Geometry check sheet. Reference: drawing and pictorial views, mm from the part's lowest x, y, z. Give positions to 0.01 mm unless a question says otherwise; leave off trailing zeros. Order: outer loops, then holes, each group sorted by start corner. A loop starts at its lowest first (then second) coordinate and runs counter-clockwise, first axis right, second up. Notation, with made-up numbers: M 68,89.25 L 110,89.25 A12 cw 110,110.25 Z; hole C 2.25,14 d3. An arc over 180 degrees is marked long. Answer as CSV lines item,"result".
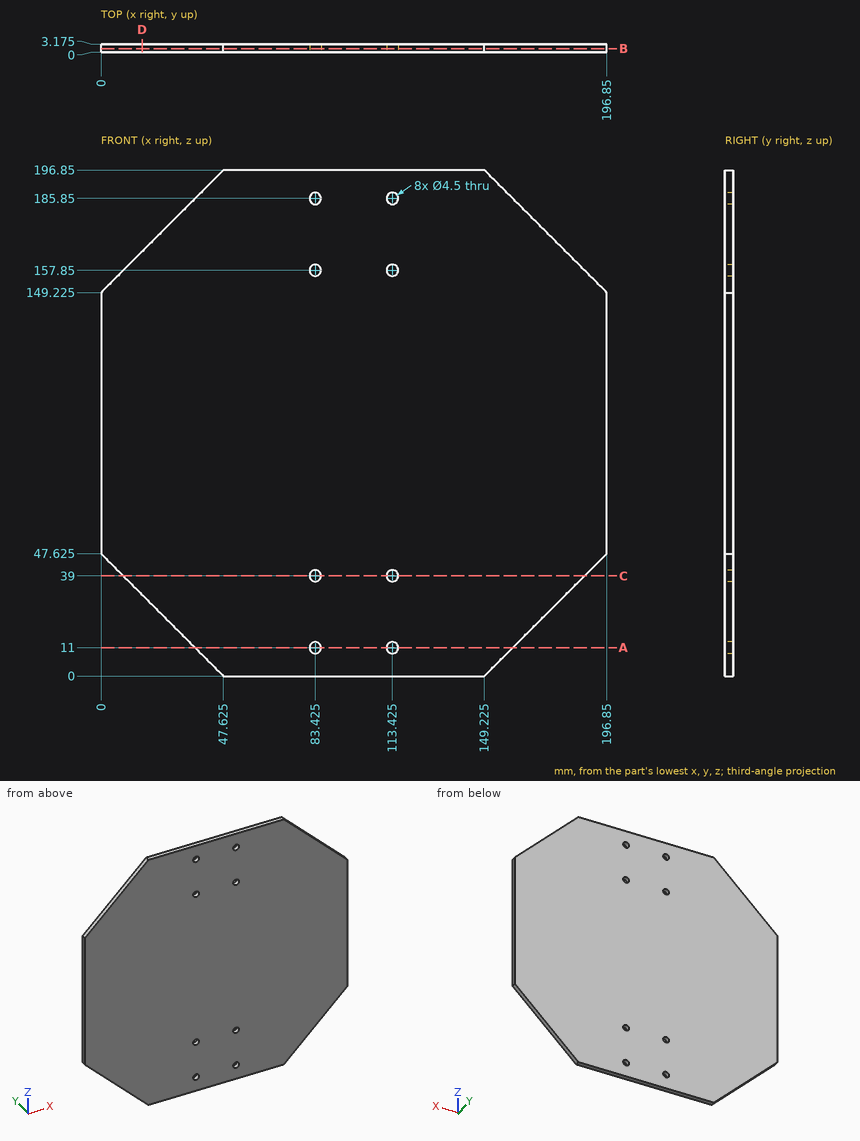
(1) Section check C-C on z = 39. Enter the section's corners in (x, y) (3 decimals).
The answers:
outline,"M 8.625,0 L 81.175,0 L 81.175,3.175 L 8.625,3.175 Z; M 85.675,0 L 111.175,0 L 111.175,3.175 L 85.675,3.175 Z; M 115.675,0 L 188.225,0 L 188.225,3.175 L 115.675,3.175 Z"
(2) Material ranges on line 1 (X direction, y = 1.6, z = 39) (3 decimals); line 2 (Z direction, x = 159, y = 1.9) (3 decimals); line 3 (Z direction, x = 32, y = 0.9) (3 decimals), recorded low to high.
The answers:
line 1,"x = 8.625 to 81.175, 85.675 to 111.175, 115.675 to 188.225"
line 2,"z = 9.775 to 187.075"
line 3,"z = 15.625 to 181.225"
(3) Section check A-A on z = 11. Enter the section's corners in (x, y) (3 decimals), then the cut area to 3 significant figures.
The answers:
outline,"M 36.625,0 L 81.175,0 L 81.175,3.175 L 36.625,3.175 Z; M 85.675,0 L 111.175,0 L 111.175,3.175 L 85.675,3.175 Z; M 115.675,0 L 160.225,0 L 160.225,3.175 L 115.675,3.175 Z"
area,"364 mm2"
(4) Gauge pin test, flat ends, axial feed: P1, Ø7, axis at x = 83.425, z = 11, coming from the -Y side; P2, Ø2.5, axis at x = 113.425, z = 157.85, coming from the -Y side. Record the tip position at first contact, or that the pin passes through.
The answers:
P1,"stops at y = 0"
P2,"passes through"
(5) Section check D-D on x = 16. Enter the section's corners in (y, z) (3 decimals), then the cut area to 3 significant figures.
The answers:
outline,"M 0,31.625 L 3.175,31.625 L 3.175,165.225 L 0,165.225 Z"
area,"424 mm2"
(6) Section check B-B on y = 1.35. State how many separate pieces and enclosed holes the cut face has, then the cut area to 3 significant figures.
The answers:
separate pieces,"1"
enclosed holes,"8"
area,"34,100 mm2"
